Autodesk Inventor part; units mm, degrees
ref_plane "YZ Plane" through (0, 0, 0) normal (1, 0, 0) x (0, 1, 0)
ref_plane "XZ Plane" through (0, 0, 0) normal (0, 1, 0) x (-1, 0, 0)
ref_plane "XY Plane" through (0, 0, 0) normal (0, 0, 1) x (1, 0, 0)
sketch "Skizze1" plane through (0, 0, 0) normal (0, 1, 0) x (-1, 0, 0)
  arc A0 (86.6025, 50) -> (86.6025, -50) centre (0, 0) ccw
  arc A1 (86.6025, 50) -> (86.6025, -50) centre (117.2454, 0) ccw
  line L0 (27.5, 90) -> (-27.5, 90)
  line L1 (-27.5, 90) -> (-27.5, 72.5)
  line L2 (-27.5, 72.5) -> (27.5, 72.5)
  line L3 (27.5, 72.5) -> (27.5, 90)
  line L4 (27.5, -72.5) -> (-27.5, -72.5)
  line L5 (-27.5, -72.5) -> (-27.5, -90)
  line L6 (-27.5, -90) -> (27.5, -90)
  line L7 (27.5, -90) -> (27.5, -72.5)
  circle A2 centre (91, 0) radius 32
  circle A3 centre (27.5, 61.5) radius 2
  circle A4 centre (-27.5, 61.5) radius 2
  circle A5 centre (27.5, -61.5) radius 2
  circle A6 centre (-27.5, -61.5) radius 2
  circle A7 centre (-75, 0) radius 11.5
  circle A8 centre (-57, 0) radius 1.5
  circle A9 centre (-93, 0) radius 1.5
  circle A10 centre (50, -15) radius 1.5
  circle A11 centre (37, -83) radius 1.5
  circle A12 centre (37, 83) radius 1.5
  circle A13 centre (-55, 70) radius 1.5
  circle A14 centre (-55, -70) radius 1.5
  point P0 (58.6025, 0)
  point P1 (27.5, -81.25)
  dimension "d0" = 100
  dimension "d1" = 100
  dimension "d2" = 17.5
  dimension "d3" = 28
  dimension "d4" = 55
  dimension "d5" = 17.5
  dimension "d7" = 72.5
  dimension "d8" = 72.5
  dimension "d9" = 27.5
  dimension "d12" = 64
  dimension "d13" = 4
  dimension "d14" = 4
  dimension "d15" = 4
  dimension "d16" = 4
  dimension "d19" = 11
  dimension "d23" = 11
  dimension "d25" = 27.5
  dimension "d26" = 27.5
  dimension "d43" = 23
  dimension "d48" = 75
  dimension "d49" = 3
  dimension "d50" = 3
  dimension "d51" = 36
  dimension "d52" = 18
  dimension "d95" = 3
  dimension "d96" = 3
  dimension "d97" = 3
  dimension "d98" = 3
  dimension "d99" = 3
  dimension "d100" = 70
  dimension "d101" = 70
  dimension "d102" = 55
  dimension "d103" = 83
  dimension "d104" = 83
  dimension "d105" = 37
  dimension "d106" = 50
  dimension "d108" = 15
extrude "Extrusion1" add sketch "Skizze1" along normal blind 4 contours A1 A0
fillet "Rundung1" radius 2 8 edges at (-27.5, 2, 72.5) (-27.5, 2, 90) (27.5, 2, 90) (27.5, 2, 72.5) (-27.5, 2, -72.5) (27.5, 2, -72.5) (27.5, 2, -90) (-27.5, 2, -90)
properties part number "base plate"
Geometry check sheet. Reference: the model listing, model coordinates, mm. Round coordinates to 2 decimals unless told otherwise and drop trailing zeros. Write each loop counter-clockwise with the first axis right and the second up, starting at its lowest first coordinate (ties: lowest second). Pieces come first, ordered by that corner, then holes.
Item 1: Section check D-D (x = 47.5). Record the boundary of the cut face in (y, z).
Determined:
outline: (0, -88) - (4, -88) - (4, 88) - (0, 88) - close
Item 2: Section check B-B (x = -69). Record the boundary of the cut face in (y, z).
Determined:
outline: (0, -72.38) - (4, -72.38) - (4, -33.34) - (0, -33.34) - close; (0, 33.34) - (4, 33.34) - (4, 72.38) - (0, 72.38) - close
Item 3: Material ranges on line 1 along X through (y, z) = (3.8, -63); line 2 along Z through (x, y) = (12, 1.3); line 3 along X through (y, z) = (2.7, 83), recorded low to high.
Determined:
line 1: x = -77.66 to -28.82, -26.18 to 26.18, 28.82 to 77.66
line 2: z = -99.28 to -90, -72.5 to 72.5, 90 to 99.28
line 3: x = -55.78 to -38.5, -35.5 to -27.5, 27.5 to 55.78
Item 4: Section check C-C (z = 42). Record the boundary of the cut face in (x, y), plus the area to 3 significant figures.
Determined:
outline: (-76.32, 0) - (90.75, 0) - (90.75, 4) - (-76.32, 4) - close
area: 668 mm2
Item 5: Mould release check, pull along X, two halves, no side actions. Record for faces 1 (the face through (-58.61, 1.97, -0.84)), 2 (the face through (8, 4, 1)), 3 (the face through (83.48, 1.97, -7.77)), 4 (the face through (99.933, 1.972, -3.664)): +X half, -X half, draft (parallel to the pull), parting line (faces both ways), or undercut.
Determined:
face 1: -X half
face 2: draft
face 3: undercut
face 4: parting line
Item 6: Section check A-A (y = 0.9). Give the number of separate pieces and of enclosed holes in the cut face, plus the area to 3 significant figures.
Determined:
separate pieces: 1
enclosed holes: 14
area: 26,100 mm2
Item 7: Go/stop test with flat-tipped pins: pin 1 Ø4 at (x, z) = (55, 70) entering from -Y; pin 2 Ø1.2 at (y, z) = (3, 80.5) entering from +X; pin 3 Ø3 at (x, z) = (-27.5, -61.5) entering from -Y. Record where each tip stops, or that it passes through.
Determined:
pin 1: stops at y = 0
pin 2: stops at x = 60.13
pin 3: passes through
